Build history of the part. All positions in model axes, mm. Face numbers are marked on the shaded views. A direction names the side the tool comes from. Round coordinates to 2 decimals unless told otherwise and drop trailing zeros. Loops run counter-clockwise (first coordinate to the right, second up) from the corner with the lowest first, then second, coordinate; pieces in that order, holes last. Notation, with made-up numbers: (71, -6.75) -> (109, -6.75) arc R30 ccw to (109, 23.25) -> close; hole circle Ø3 at (81.25, 31.5). An arc over 180 degrees is marked (long way). Put each result on its own line as item: value. Start each with the question number.
Item 1: Tool access for the marked faces 5, 6 and 7: list every direction of +Z, -Z, +X, -X, +Y, -Y with a clear straight run to the whole face (end or side of a thin tool).
Item 2: Cut at A-A, the plane y = -29. List the corners of the cut face in (x, z).
Item 3: Pull direction Y, two halves, no side cores. Call the marked faces 1, 2, 3 and 4: +Y half, -Y half, draft (parallel to the pull), parting line (faces both ways), or undercut.
Item 4: Drill centre lines: probe 1 along X at (y, z) = (-25.5, 12); probe 2 along Y at (x, z) = (-30, -0.5). Where is each one in solid material? Low to high. Write a range as [from, to].
Item 5: Cut at D-D, the plane y = -3. List the corners of the cut face in (x, z).
Item 6: Flat gauge pins, fed straight in: pin 1 Ø1.6 at (x, z) = (-28, -1) entering from -Y; pin 2 Ø1.6 at (y, z) = (-24.5, -1) entering from +X; pin 3 Ø24 at (x, y) = (-1.5, 14) entering from -Z. Where does each tip first touch, or does it go through?
Item 7: Cut at C-C, the plane z = 3.75. List the corners of the cut face in (x, y).
```python
from build123d import *

# Parameters (mm, degrees)
F0_W      = 79.8
F0_H      = 79.8
F1_DEPTH  = 15
F2_W      = 74
F2_H      = 74
F3_DEPTH  = 13
F4_W      = 73.8
F4_H      = 73.8
F4_W_2    = 69.8
F4_H_2    = 69.8
F5_DEPTH  = 2
F7_DEPTH  = 2
F8_R      = 2
F9_R      = 4
F10_R     = 0.99999
F12_DEPTH = 79.801
F13_R     = 5
F14_R     = 4
F15_R     = 1


# Not quite as in the source:
# - a fillet or chamfer is up to 0.001 mm smaller than in the source, because OpenCascade refuses the exact size


with BuildPart() as f1:
    # F0 (on Top) → F1 (new body)
    with BuildSketch(Plane.XY):
        Rectangle(F0_W, F0_H)
    extrude(amount=F1_DEPTH)

    # F2 (on face) → F3 (cut)
    with BuildSketch(Plane.XY.offset(15)):
        Rectangle(F2_W, F2_H)
    extrude(amount=-F3_DEPTH, mode=Mode.SUBTRACT)

    # F4 (on face) → F5 (join)
    with BuildSketch(Plane(origin=(0, 0, 0), x_dir=(1, 0, 0), z_dir=(0, 0, -1))):
        Rectangle(F4_W, F4_H)
        Rectangle(F4_W_2, F4_H_2, mode=Mode.SUBTRACT)
    extrude(amount=F5_DEPTH)

    # F6 (on face) → F7 (cut, through all)
    with BuildSketch(Plane(origin=(0, 0, -2), x_dir=(1, 0, 0), z_dir=(0, 0, -1))):
        Polygon((36.9, -21.9), (36.9, 21.9), (21.9, 21.9), (21.9, 36.9), (-21.9, 36.9), (-21.9, 21.9), (-36.9, 21.9), (-36.9, -21.9), (-21.9, -21.9), (-21.9, -36.9), (21.9, -36.9), (21.9, -21.9), align=None)
    extrude(amount=-F7_DEPTH, mode=Mode.SUBTRACT)

    # F8
    f8_edges = [f1.edges().sort_by_distance(p)[0] for p in [
        (-34.9, 34.9, -1),
        (-34.9, -34.9, -1),
        (34.9, -34.9, -1),
        (34.9, 34.9, -1),
    ]]
    fillet(f8_edges, radius=F8_R)

    # F9
    f9_edges = [f1.edges().sort_by_distance(p)[0] for p in [
        (-36.9, 36.9, -1),
        (36.9, 36.9, -1),
        (36.9, -36.9, -1),
        (-36.9, -36.9, -1),
    ]]
    fillet(f9_edges, radius=F9_R)

    # F10 (radius 1 in the source; OpenCascade refuses exactly that, so slightly less here)
    f10_edges = [f1.edges().sort_by_distance(p)[0] for p in [
        (21.9, -35.9, -2),
        (21.9, -35.9, 0),
        (35.9, -21.9, -2),
        (35.9, -21.9, 0),
        (-35.9, -21.9, -2),
        (-35.9, -21.9, 0),
        (-21.9, -35.9, -2),
        (-21.9, -35.9, 0),
        (-35.9, 21.9, -2),
        (-35.9, 21.9, 0),
        (-21.9, 35.9, -2),
        (-21.9, 35.9, 0),
        (21.9, 35.9, -2),
        (21.9, 35.9, 0),
        (35.9, 21.9, -2),
        (35.9, 21.9, 0),
    ]]
    fillet(f10_edges, radius=F10_R)

    # F11 (on face) → F12 (cut, through all)
    with BuildSketch(Plane.XZ.offset(39.9)):
        Polygon((20, 15), (-20, 15), (-16.3888888889, 2), (16.3888888889, 2), align=None)
    extrude(amount=-F12_DEPTH, mode=Mode.SUBTRACT)

    # F13
    f13_edges = [f1.edges().sort_by_distance(p)[0] for p in [
        (-20, -38.45, 15),
        (-16.388889, -38.45, 2),
        (16.388889, -38.45, 2),
        (20, -38.45, 15),
        (16.388889, 38.45, 2),
        (20, 38.45, 15),
        (-20, 38.45, 15),
        (-16.388889, 38.45, 2),
    ]]
    fillet(f13_edges, radius=F13_R)

    # F14
    f14_edges = [f1.edges().sort_by_distance(p)[0] for p in [
        (39.9, -39.9, 7.5),
        (39.9, 39.9, 7.5),
        (-39.9, -39.9, 7.5),
        (-39.9, 39.9, 7.5),
    ]]
    fillet(f14_edges, radius=F14_R)

    # F15
    f15_edges = [f1.edges().sort_by_distance(p)[0] for p in [
        (37, 37, 8.5),
        (-37, 37, 8.5),
        (-37, -37, 8.5),
        (37, -37, 8.5),
    ]]
    fillet(f15_edges, radius=F15_R)


solid = f1.part
```
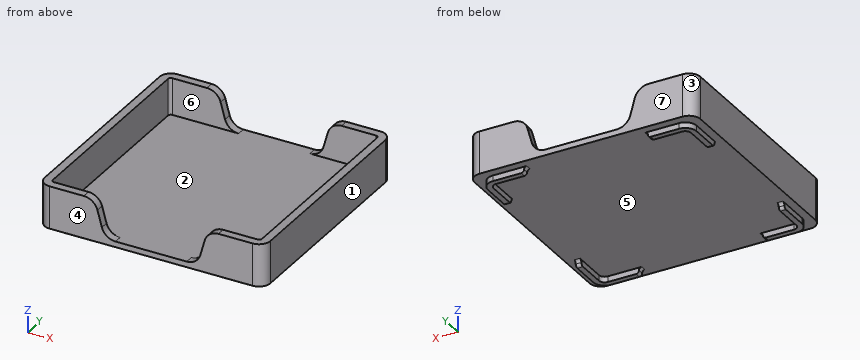
Reply:
1. face 5: -Z
1. face 6: +Z
1. face 7: +Z, -Z, +X, -X, +Y
2. outline: (-39.9, 0) -> (-36.9, 0) -> (-36.9, -2) -> (-34.9, -2) -> (-34.9, 0) -> (34.9, 0) -> (34.9, -2) -> (36.9, -2) -> (36.9, 0) -> (39.9, 0) -> (39.9, 15) -> (37, 15) -> (37, 2) -> (-37, 2) -> (-37, 15) -> (-39.9, 15) -> close
3. face 1: draft
3. face 2: undercut
3. face 3: +Y half
3. face 4: -Y half
4. probe 1: x = [-39.9, -37], [37, 39.9]
4. probe 2: y = [-36.9, -34.9], [34.9, 36.9]
5. outline: (-39.9, 0) -> (39.9, 0) -> (39.9, 15) -> (37, 15) -> (37, 2) -> (-37, 2) -> (-37, 15) -> (-39.9, 15) -> close
6. pin 1: stops at y = -36.9
6. pin 2: stops at x = 36.9
6. pin 3: stops at z = 0
7. outline: (-39.9, -35.9) arc R4 ccw to (-35.9, -39.9) -> (-16.39, -39.9) -> (-16.39, -37) -> (-36, -37) arc R1 cw to (-37, -36) -> (-37, 36) arc R1 cw to (-36, 37) -> (-16.39, 37) -> (-16.39, 39.9) -> (-35.9, 39.9) arc R4 ccw to (-39.9, 35.9) -> close; (16.39, -39.9) -> (35.9, -39.9) arc R4 ccw to (39.9, -35.9) -> (39.9, 35.9) arc R4 ccw to (35.9, 39.9) -> (16.39, 39.9) -> (16.39, 37) -> (36, 37) arc R1 cw to (37, 36) -> (37, -36) arc R1 cw to (36, -37) -> (16.39, -37) -> close
